Design review of the part built by this model. Coordinates are the model's own, in mm. A direction names the side the tool comes from. Give positions to 0.01 mm unless a question says otherwise; leave off trailing zeros. Answer as a JSON object with one key per item and string values.
```python
from build123d import *

# Parameters (mm, degrees)
SKETCH1_W           = 127
SKETCH1_H           = 95.25
BOSS_EXTRUDE1_DEPTH = 6.35
SKETCH2_R           = 3.96875
CUT_EXTRUDE1_DEPTH  = 7.35
SKETCH3_W           = 6.35
SKETCH3_H           = 12.7
CUT_EXTRUDE2_DEPTH  = 7.35
SKETCH4_W           = 6.35
SKETCH4_H           = 12.7
CUT_EXTRUDE3_DEPTH  = 7.35
LPATTERN1_COUNT     = 4
LPATTERN1_PITCH     = 25.4
CUT_EXTRUDE4_DEPTH  = 7.35
LPATTERN2_COUNT     = 4
LPATTERN2_PITCH     = 25.4


with BuildPart() as part:
    # Sketch1 → Boss-Extrude1 (new body)
    with BuildSketch(Plane.XY):
        with Locations((63.5, 47.625)):
            Rectangle(SKETCH1_W, SKETCH1_H)
    extrude(amount=BOSS_EXTRUDE1_DEPTH)

    # Sketch2 → Cut-Extrude1 (cut, through all)
    with BuildSketch(Plane.XY.offset(6.35)):
        with Locations((63.5, 38.1)):
            Circle(SKETCH2_R)
    extrude(amount=-CUT_EXTRUDE1_DEPTH, mode=Mode.SUBTRACT)

    # Sketch3 → Cut-Extrude2 (cut, through all)
    with BuildSketch(Plane.XY.offset(6.35)):
        with Locations((3.175, 19.05)):
            Rectangle(SKETCH3_W, SKETCH3_H)
    cut_extrude2 = extrude(amount=-CUT_EXTRUDE2_DEPTH, mode=Mode.SUBTRACT)

    # Sketch4 → Cut-Extrude3 (cut, through all)
    with BuildSketch(Plane.XY.offset(6.35)):
        with Locations((123.825, 19.05)):
            Rectangle(SKETCH4_W, SKETCH4_H)
    cut_extrude3 = extrude(amount=-CUT_EXTRUDE3_DEPTH, mode=Mode.SUBTRACT)

    # LPattern1: Cut-Extrude2, Cut-Extrude3 ×4
    with Locations(*[(0, i * LPATTERN1_PITCH, 0) for i in range(1, LPATTERN1_COUNT)]):
        add(cut_extrude2, mode=Mode.SUBTRACT)
        add(cut_extrude3, mode=Mode.SUBTRACT)

    # Sketch5 → Cut-Extrude4 (cut, through all)
    with BuildSketch(Plane.XY.offset(6.35)):
        Polygon((102.338352728, 40.824853058), (104.768392524, 34.958218027), (110.635027555, 37.388257822), (108.20498776, 43.254892854), align=None)
        Polygon((109.628472115, 23.224947964), (107.198432319, 29.091582995), (113.065067351, 31.521622791), (115.495107146, 25.65498776), align=None)
    cut_extrude4 = extrude(amount=-CUT_EXTRUDE4_DEPTH, mode=Mode.SUBTRACT)

    # LPattern2: Cut-Extrude4 ×4
    with Locations(*[Vector(-0.923879533, -0.382683432, 0) * (i * LPATTERN2_PITCH) for i in range(1, LPATTERN2_COUNT)]):
        add(cut_extrude4, mode=Mode.SUBTRACT)


solid = part.part
```
(1) For line 1 along X through (y, z) = (30, 0.75); line 2 along X through (y, z) = (6.5, 5.5); line 3 along Y through (x, z) = (63.5, 2), list the stretches that pass through material, from the lowest coordinate up.
Here are the results:
{"line 1": "x = 0 to 79.33, 86.2 to 109.39, 113.7 to 127", "line 2": "x = 0 to 34.08, 36.06 to 61.57, 68.44 to 127", "line 3": "y = 0 to 4.12, 10.99 to 17.86, 18.44 to 34.13, 42.07 to 95.25"}
(2) For faces 1 (the flat face through (81.85, 32.34, 3.22)), 2 (the flat face through (124, 63.5, 3)), 3 (the flat face through (39.775, 1.164, 3.219)), 4 (the flat face through (63, 48, 6.35)), list the 3-axis set-ups (+Z, -Z, +X, -X, +Y, -Y) from which the entire face can be reached by the end or side of a thin tool; tool diameter is ignored.
Here are the results:
{"face 1": "+Z, -Z", "face 2": "+Z, -Z, +X", "face 3": "+Z, -Z, -Y", "face 4": "+Z, +X, -X, +Y, -Y"}
(3) We need section A-A, the plane z = 1. Give the number of separate pieces and of enclosed holes in the cut face, then the cut area to 3 significant figures.
Here are the results:
{"separate pieces": "1", "enclosed holes": "8", "area": "11,200 mm²"}
(4) Clearance check with flat-ended pins moving along their axes: pin 1 (3 mm diameter, centred on y = 46.5, z = 1.5, fed in from +X); pin 2 (1.9 mm diameter, centred on y = 41.5, z = 2, fed in from -X); pin 3 (1.9 mm diameter, centred on x = 3, z = 4, fed in from +Y). State where each tip first meets the part, or that it passes through.
Here are the results:
{"pin 1": "stops at x = 120.65", "pin 2": "stops at x = 6.35", "pin 3": "stops at y = 88.9"}
(5) The part is to be moulded in two halves that separate along Y. For faces 5 (the flat face through (18, 0, 3)), 6 (the flat face through (63, 48, 0)), 7 (the flat face through (120.65, 70, 3)), say which applies: +Y half, -Y half, draft (parallel to the pull), parting line (faces both ways), or undercut.
Here are the results:
{"face 5": "-Y half", "face 6": "draft", "face 7": "undercut"}
